Could you check a few things on this model? Use its own coordinates, in mm. A direction names the side the tool comes from. Coordinates: 2 decimals unless noted, no trailing zeros. Use a Markdown table: item, result. Add a question column.
1) Will these pins go through, and if not, where does the flat tip stop? pin 1 Ø4.5 at (x, y) = (25, -13.5) entering from -Z; pin 2 Ø8 at (x, y) = (-25, 13.5) entering from -Z; pin 3 Ø3 at (x, z) = (43.5, 1.5) entering from +Y; pin 4 Ø10.5 at (x, y) = (40, 0) entering from +Z.
2) Thinking about a two-plate mould opening in X: for faces 3 (the flat face through (16, 1, 12.7)), 4 (the cylindrical face through (-22.253, -13.621, 8.65)), 5 (the cylindrical face through (-36.8, -2.4, 6.3)), 6 (the cylindrical face through (-9.764, 74.362, 6.268)), which applies, +X half, -X half, draft (parallel to the pull), parting line (faces both ways), or undercut?
3) Which directions (+Z, -Z, +X, -X, +Y, -Y) give clear straight access to the entire face, cutting with the end or side of a thin tool? Please do faces 1 (the cylindrical face through (-29.87, 13.29, 2.72)), 2 (the cylindrical face through (43.2, -2.4, 6.3)).
4) If I drill on L1, parallel to Y at x = -27.5, z = 5.5; L2, parallel to X at y = 13.5, z = 7.5 (3 decimals); L3, parallel to Y at x = 23.5, z = 6.5, over which ranges is the centre line in solid material (lowest first)? Write a range as [from, to].
5) If we section it at A-A (z = 9.25): Give the number of separate pieces and of enclosed holes in the cut face, plus the area to 3 significant figures.
```python
from build123d import *

# Parameters (mm, degrees)
F0_R           = 75
F1_DEPTH       = 12.7
F2_D           = 5.5
F2_CBORE_D     = 9.75
F2_CBORE_DEPTH = 5
F4_D           = 7
F5_D           = 7.9375
F6_SIZE        = 0.5
F8_D           = 8


# Not quite as in the source:
# - a length typed as a fraction of an inch, garbled in the dataset ("3 / 203.2 mm" for 3/8 in), is restored


with BuildPart() as f1:
    # F0 (on Top) → F1 (new body)
    with BuildSketch(Plane.XY):
        Circle(F0_R)
    extrude(amount=F1_DEPTH)

    # F2 (through all)
    with Locations(Plane(origin=(0, 0, 0), x_dir=(1, 0, 0), z_dir=(0, 0, -1))):
        with Locations((-25, 13.5), (25, 13.5), (-25, -13.5), (25, -13.5)):
            CounterBoreHole(F2_D / 2, F2_CBORE_D / 2, F2_CBORE_DEPTH)

    # F4 (through all)
    with Locations(Plane.XY.offset(12.7)):
        with Locations((0, 61), (58, 18.8), (-58, 18.8), (-35.8, -49.3), (35.8, -49.3)):
            Hole(F4_D / 2)

    # F5 (through all)
    with Locations(Plane(origin=(0, 0, 0), x_dir=(1, 0, 0), z_dir=(0, 0, -1))):
        with Locations((0, 0)):
            Hole(F5_D / 2)

    # F6
    f6_edges = [f1.edges().sort_by_distance(p)[0] for p in [
        (-75, 0, 0),
        (-39.3, -49.3, 0),
        (-29.875, -13.5, 0),
        (32.3, -49.3, 0),
        (20.125, -13.5, 0),
        (-3.96875, 0, 0),
        (-61.5, 18.8, 0),
        (-29.875, 13.5, 0),
        (20.125, 13.5, 0),
        (54.5, 18.8, 0),
        (-3.5, 61, 0),
        (-75, 0, 12.7),
        (-39.3, -49.3, 12.7),
        (-27.75, -13.5, 12.7),
        (32.3, -49.3, 12.7),
        (22.25, -13.5, 12.7),
        (-3.96875, 0, 12.7),
        (-61.5, 18.8, 12.7),
        (-27.75, 13.5, 12.7),
        (22.25, 13.5, 12.7),
        (54.5, 18.8, 12.7),
        (-3.5, 61, 12.7),
    ]]
    chamfer(f6_edges, length=F6_SIZE)

    # F8 (through all)
    with Locations(Plane.XY.offset(12.7)):
        with Locations((-40, 0), (40, 0)):
            Hole(F8_D / 2)


solid = f1.part
```
Answer sheet:
| question | item | result |
|---|---|---|
| 1 | pin 1 | through |
| 1 | pin 2 | z = 5 |
| 1 | pin 3 | y = 62.14 |
| 1 | pin 4 | z = 12.7 |
| 2 | face 3 | draft |
| 2 | face 4 | undercut |
| 2 | face 5 | undercut |
| 2 | face 6 | parting line |
| 3 | face 1 | -Z |
| 3 | face 2 | +Z, -Z |
| 4 | L1 | [-69.78, -14.65], [-12.35, 12.35], [14.65, 69.78] |
| 4 | L2 | [-73.775, -27.75], [-22.25, 22.25], [27.75, 73.775] |
| 4 | L3 | [-71.22, -15.8], [-11.2, 11.2], [15.8, 71.22] |
| 5 | separate pieces | 1 |
| 5 | enclosed holes | 12 |
| 5 | area | 17,200 mm2 |
